The figure shows three views and two pictorial views of one solid part (mm, origin at its lowest corner). Answer the questions. A direction names the side the tool comes from. Coordinates: 2 decimals unless noted, no trailing zeros. Write each loop counter-clockwise with the first axis right and the second up, starting at its lowest first coordinate (ties: lowest second). Pieces come first, ordered by that corner, then holes.
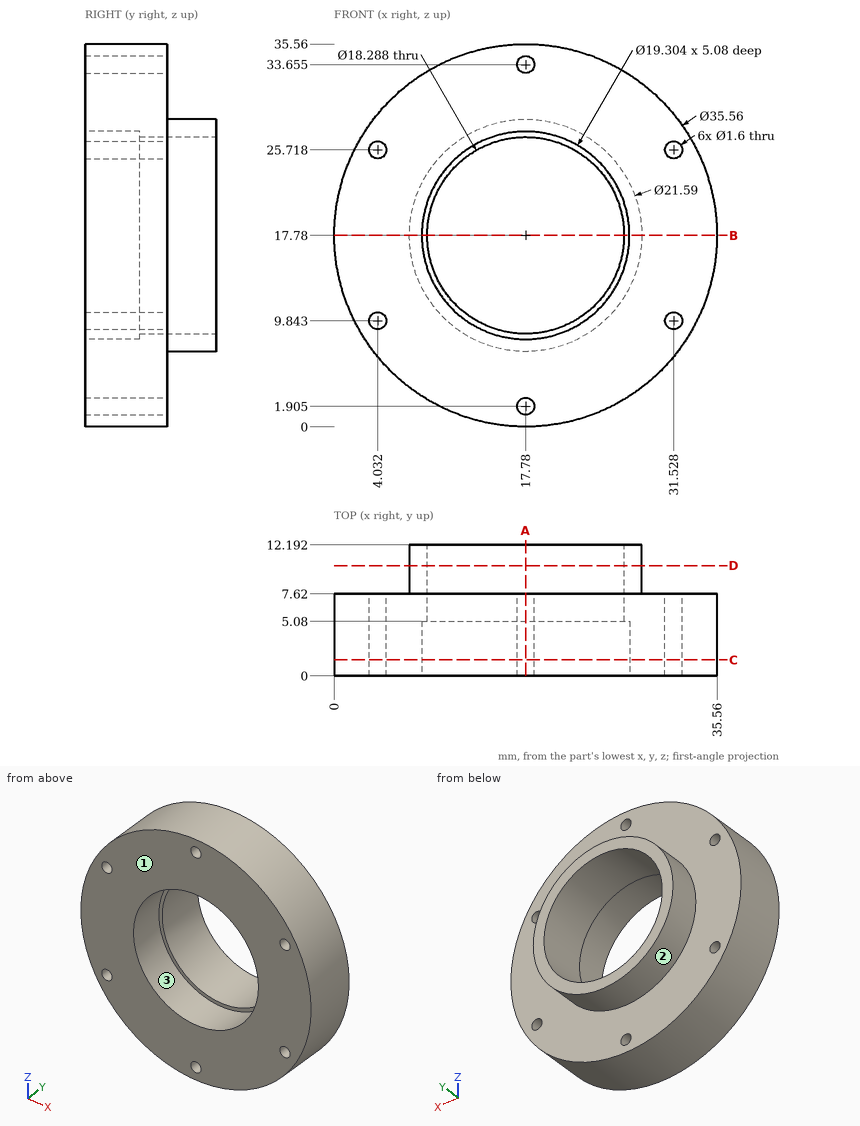
Item 1: Given pin 1 (5 mm diameter, centred on y = 4, z = 24, fed in from -X); pin 2 (1.3 mm diameter, centred on x = 31.53, z = 25.72, fed in from +Y); pin 3 (2 mm diameter, centred on x = 16.5, y = 3.5, fed in from -Z); pin 4 (2.5 mm diameter, centred on x = 17.78, z = 33.655, fed in from +Y), each flat-ended and moving along its own axis, determine where each tip first touches the part or whether it passes through.
Item 2: The part is cut by section D-D (y = 10.25). Give the vertices of the cut face in (x, z) (1 decimal).
Item 3: Find the intervals of material crossed by probe 1 along Z at (x, y) = (17.78, 2.25) (1 decimal); probe 2 along Y at (x, z) = (25, 26.5); probe 3 along Z at (x, y) = (21, 2.75) (1 decimal), in increasing order.
Item 4: For the marked faces 1, 2 and 3, determine the directions among +Z, -Z, +X, -X, +Y, -Y from which every point of the face is accessible in a straight line to the end or side of a thin tool.
Item 5: The part is cut by section C-C (y = 1.5). Give the vertices of the cut face in (x, z) (1 decimal).
Item 6: The part is cut by section B-B (z = 17.78). Give the vertices of the cut face in (x, y) (1 decimal).
Item 7: The part is cut by section A-A (x = 17.78). Give the vertices of the cut face in (y, z) (1 decimal), and give its area (3 significant figures).
Answer:
1. pin 1: stops at x = 0.39
1. pin 2: passes through
1. pin 3: stops at z = 0
1. pin 4: stops at y = 7.62
2. outline: circle Ø21.6 at (17.8, 17.8); hole circle Ø18.3 at (17.8, 17.8)
3. probe 1: z = 0 to 1.1, 2.7 to 8.1, 27.4 to 32.9, 34.5 to 35.6
3. probe 2: y = 0 to 7.62
3. probe 3: z = 0.3 to 8.7, 26.9 to 35.3
4. face 1: +Z, -Z, +X, -X, -Y
4. face 2: +Y
4. face 3: -Y
5. outline: circle Ø35.6 at (17.8, 17.8); hole circle Ø1.6 at (4, 9.8); hole circle Ø1.6 at (4, 25.7); hole circle Ø19.3 at (17.8, 17.8); hole circle Ø1.6 at (17.8, 1.9); hole circle Ø1.6 at (17.8, 33.7); hole circle Ø1.6 at (31.5, 9.8); hole circle Ø1.6 at (31.5, 25.7)
6. outline: (0, 0) - (8.1, 0) - (8.1, 5.1) - (8.6, 5.1) - (8.6, 12.2) - (7, 12.2) - (7, 7.6) - (0, 7.6) - close; (26.9, 5.1) - (27.4, 5.1) - (27.4, 0) - (35.6, 0) - (35.6, 7.6) - (28.6, 7.6) - (28.6, 12.2) - (26.9, 12.2) - close
7. outline: (0, 0) - (7.6, 0) - (7.6, 1.1) - (0, 1.1) - close; (0, 2.7) - (7.6, 2.7) - (7.6, 7) - (12.2, 7) - (12.2, 8.6) - (5.1, 8.6) - (5.1, 8.1) - (0, 8.1) - close; (0, 27.4) - (5.1, 27.4) - (5.1, 26.9) - (12.2, 26.9) - (12.2, 28.6) - (7.6, 28.6) - (7.6, 32.9) - (0, 32.9) - close; (0, 34.5) - (7.6, 34.5) - (7.6, 35.6) - (0, 35.6) - close
7. area: 117 mm2
